```python
from build123d import *

# Parameters (mm, degrees)
SKETCH2_W                      = 146.05
SKETCH2_H                      = 44.45
BOSS_EXTRUDE1_DEPTH            = 12.7
F_1_4_20_TAPPED_HOLE1_D        = 5.1054
F_8_32_TAPPED_HOLE1_AT_2_COUNT = 2
F_8_32_TAPPED_HOLE1_AT_2_PITCH = 31.75


with BuildPart() as part:
    # Sketch2 → Boss-Extrude1 (new body)
    with BuildSketch(Plane(origin=(0, 0, 0), x_dir=(1, 0, 0), z_dir=(0, 1, 0))):
        Rectangle(SKETCH2_W, SKETCH2_H)
    extrude(amount=BOSS_EXTRUDE1_DEPTH)

    # 1/4-20 Tapped Hole1 (through all)
    with Locations(Plane(origin=(0, 0, 0), x_dir=(-1, 0, 0), z_dir=(0, -1, 0))):
        with Locations((0, 0)):
            Hole(F_1_4_20_TAPPED_HOLE1_D / 2)

    # Sketch7 → #8-32 Tapped Hole1 (revolve, cut)
    with BuildSketch(Plane(origin=(-73.025, 6.35, -15.875), x_dir=(0, 0, 1), z_dir=(0, 1, 0))):
        Polygon((0, 0), (0, 7.387806461), (1.7272, 6.35), (1.7272, 0), align=None)
    f_8_32_tapped_hole1 = revolve(axis=Axis((-79.375, 6.35, -15.875), (1, 0, 0)), mode=Mode.SUBTRACT)

    # #8-32 Tapped Hole1 at 2: #8-32 Tapped Hole1 ×2
    with Locations(*[(0, 0, i * F_8_32_TAPPED_HOLE1_AT_2_PITCH) for i in range(1, F_8_32_TAPPED_HOLE1_AT_2_COUNT)]):
        add(f_8_32_tapped_hole1, mode=Mode.SUBTRACT)

    # Mirror1: #8-32 Tapped Hole1 across plane
    add(f_8_32_tapped_hole1.mirror(Plane(origin=(0, 0, 0), x_dir=(0, 0, 1), z_dir=(1, 0, 0))), mode=Mode.SUBTRACT)

    # Mirror1 copy 1 sketch → Mirror1 copy 1 (revolve, cut)
    with BuildSketch(Plane(origin=(73.025, 6.35, 15.875), x_dir=(0, 0, 1), z_dir=(0, 1, 0))):
        Polygon((0, 0), (0, -7.387806461), (1.7272, -6.35), (1.7272, 0), align=None)
    revolve(axis=Axis((79.375, 6.35, 15.875), (1, 0, 0)), mode=Mode.SUBTRACT)


solid = part.part
```
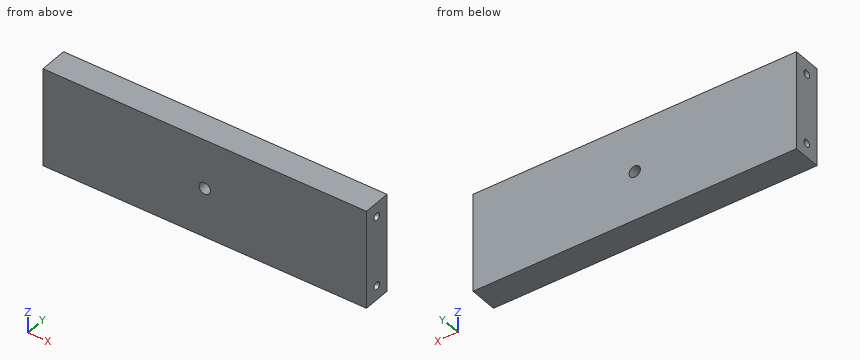
The listing builds one solid part. Answer for the finished solid, in the listing's coordinates (mm). Round coordinates to 2 decimals unless told otherwise and drop trailing zeros. Order: outer loops, then holes, each group sorted by start corner. A loop starts at its lowest first (then second) coordinate and runs counter-clockwise, first axis right, second up. Notation, with made-up numbers: (38.5, 66.5) - (79.5, 66.5) arc R21 cw to (79.5, 73.5) - close; hole circle Ø7 at (0, 64.5). An arc over 180 degrees is marked (long way). Put each result on its own line as item: value. Start each with the question number.
(1) Given P1, Ø3, axis at y = 6.35, z = 15.875, coming from the -X side; P2, Ø2, axis at y = 6.35, z = -15.875, coming from the +X side, each flat-ended and moving along its own axis, determine where each tip first touches the part or whether it passes through.
(2) Find section B-B (x = 0). Give the vertices of the cut face in (y, z) (3 decimals), plus the area to 3 significant figures.
(3) Find section A-A (z = 0). Give the vertices of the cut face in (x, y) (3 decimals), plus the area to 3 significant figures.
(4) Straight lines are drawn through the part: probe 1 along Z at (x, y) = (-69.25, 6.35) (3 decimals); probe 2 along X at (y, z) = (8.5, -1.5) (1 decimal). For each, find the intervals that lie inside material, in ascending order. Write a range as from..to.
Reply:
1. P1: x = -66.54
1. P2: x = 66.24
2. outline: (0, -22.225) - (12.7, -22.225) - (12.7, -2.553) - (0, -2.553) - close; (0, 2.553) - (12.7, 2.553) - (12.7, 22.225) - (0, 22.225) - close
2. area: 500 mm^2
3. outline: (-73.025, 0) - (-2.553, 0) - (-2.553, 12.7) - (-73.025, 12.7) - close; (2.553, 0) - (73.025, 0) - (73.025, 12.7) - (2.553, 12.7) - close
3. area: 1,790 mm^2
4. probe 1: -22.225..-17.602, -14.148..14.148, 17.602..22.225
4. probe 2: -73..-2.1, 2.1..73
